Drawing for the job (mm, zero at the part's lowest x, y, z). Coordinates: 2 decimals unless noted, no trailing zeros. Write each loop counter-clockwise with the first axis right and the second up, starting at its lowest first coordinate (ties: lowest second). Pieces come first, ordered by that corner, then holes. Notation, with made-up numbers: (15.25, -1.75) - (31.25, -1.75) arc R12 ccw to (31.25, 2.25) - close; hole circle Ø3 at (75, 46.25). An arc over 180 degrees is marked (long way). Write each question's results on one line, items separated by ' | '.
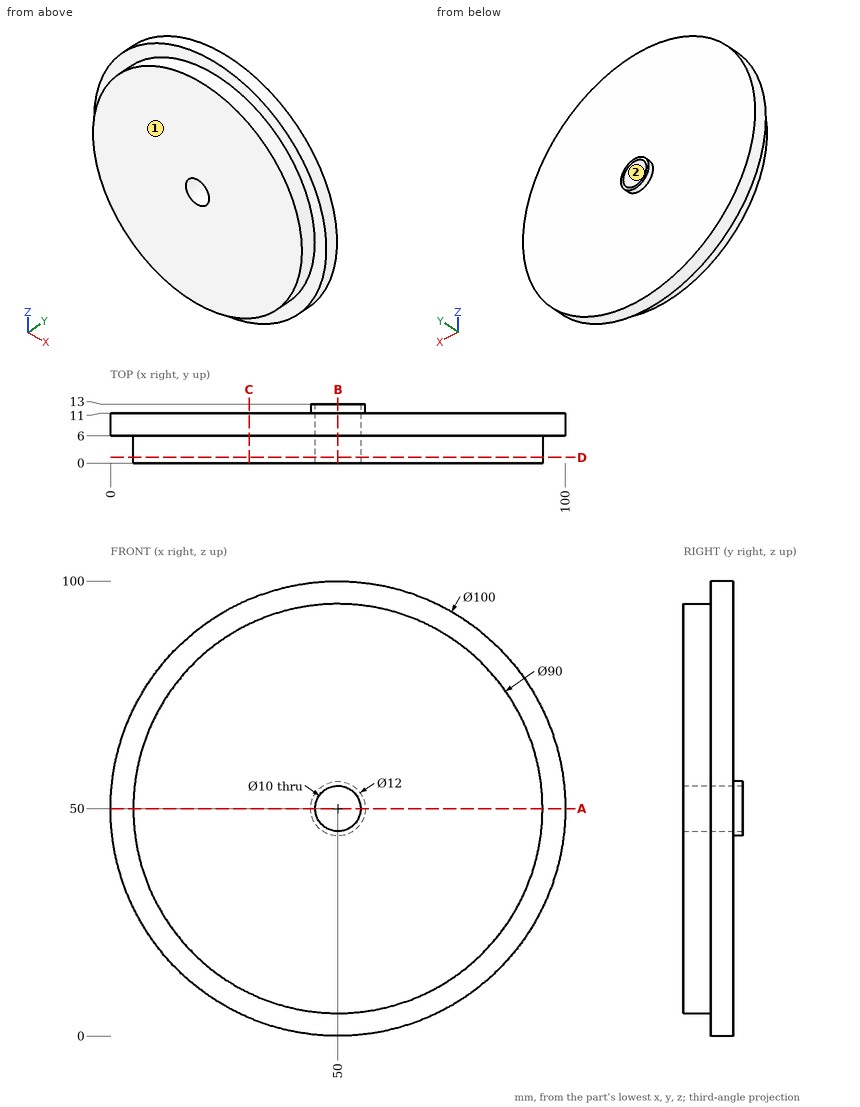
(1) Saw through at A-A on z = 50. Write the cut outline in (x, y).
Return value:
outline: (0, 6) - (5, 6) - (5, 0) - (45, 0) - (45, 13) - (44, 13) - (44, 11) - (0, 11) - close; (55, 0) - (95, 0) - (95, 6) - (100, 6) - (100, 11) - (56, 11) - (56, 13) - (55, 13) - close
(2) Saw through at B-B on x = 50. Write the cut outline in (y, z).
Return value:
outline: (0, 5) - (6, 5) - (6, 0) - (11, 0) - (11, 44) - (13, 44) - (13, 45) - (0, 45) - close; (0, 55) - (13, 55) - (13, 56) - (11, 56) - (11, 100) - (6, 100) - (6, 95) - (0, 95) - close
(3) Saw through at C-C on x = 30.5. Write the cut outline in (y, z).
Return value:
outline: (0, 9.44) - (6, 9.44) - (6, 3.96) - (11, 3.96) - (11, 96.04) - (6, 96.04) - (6, 90.56) - (0, 90.56) - close
(4) Wall check: line 1 (Z direction, x = 50, y = 10.5); line 2 (Z direction, x = 50, y = 3.5); line 3 (Y direction, x = 64.5, z = 35.5). Give the ranges that are in metal, low to high. Write a range as from..to.
Return value:
line 1: z = 0..45, 55..100 | line 2: z = 5..45, 55..95 | line 3: y = 0..11
(5) Saw through at D-D on y = 1.25. Write the cut outline in (x, z), then the cut area to 3 significant figures.
Return value:
outline: circle Ø90 at (50, 50); hole circle Ø10 at (50, 50) | area: 6,280 mm^2
(6) Flat gauge pins, fed straight in: P1, Ø3, axis at y = 6, z = 76, coming from the -X side; P2, Ø4, axis at x = 85, z = 33.5, coming from the +Y side; P3, Ø2, axis at y = 6.5, z = 32, coming from the -X side. Where does each tip first touch, or does it go through?
Return value:
P1: stops at x = 6.41 | P2: stops at y = 11 | P3: stops at x = 2.98
(7) Two-plate mould, pull along Z, no slides. Class the marked faces 1 and 2: released by +Z, released by -Z, zero draft, split by the parting line, or undercut.
Return value:
face 1: zero draft | face 2: undercut
